For this review, use the dimensioned drawing (mm, ordinates from the lowest corner) and the shaded views. A direction names the side the tool comes from. Round coordinates to 2 decimals unless told otherwise and drop trailing zeros. Write each loop counter-clockwise with the first axis right and the second up, starting at its lowest first coordinate (ties: lowest second). Pieces come first, ordered by that corner, then holes.
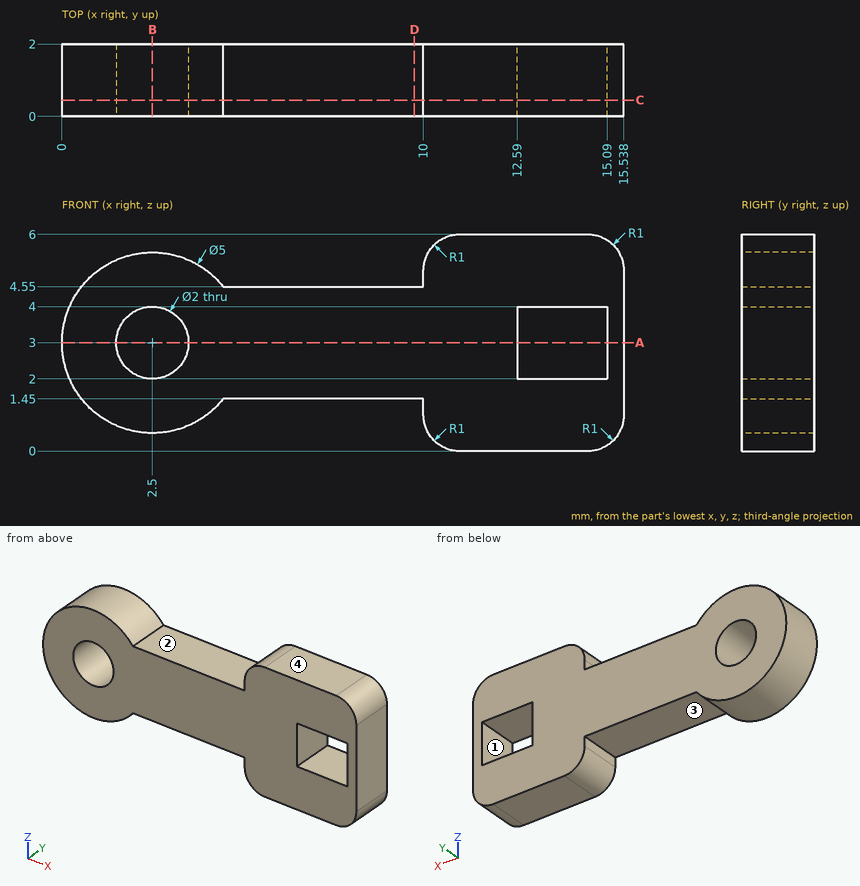
(1) We need section B-B, the plane x = 2.5. Give the boundary of the cut face in (y, z).
Geometry check:
outline: (0, 0.5) - (2, 0.5) - (2, 2) - (0, 2) - close; (0, 4) - (2, 4) - (2, 5.5) - (0, 5.5) - close
(2) For line 1 along X through (y, z) = (1.55, 3); line 2 along Z through (x, y) = (13, 0.5); line 3 along X through (y, z) = (1.75, 2.25) (1 decimal), list the stretches that pass through material, from the lowest coordinate up.
Geometry check:
line 1: x = 0 to 1.5, 3.5 to 12.59, 15.09 to 15.54
line 2: z = 0 to 2, 4 to 6
line 3: x = 0.1 to 1.8, 3.2 to 12.6, 15.1 to 15.5
(3) We need section D-D, the plane x = 9.75. Give the boundary of the cut face in (y, z).
Geometry check:
outline: (0, 1.45) - (2, 1.45) - (2, 4.55) - (0, 4.55) - close
(4) We need section C-C, the plane y = 0.45. Give the boundary of the cut face in (x, z).
Geometry check:
outline: (4.46, 1.45) - (10, 1.45) - (10, 1) arc R1 ccw to (11, 0) - (14.54, 0) arc R1 ccw to (15.54, 1) - (15.54, 5) arc R1 ccw to (14.54, 6) - (11, 6) arc R1 ccw to (10, 5) - (10, 4.55) - (4.46, 4.55) arc R2.5 ccw (long way) to start; hole circle Ø2 at (2.5, 3); hole (12.59, 2) - (15.09, 2) - (15.09, 4) - (12.59, 4) - close
(5) For pin 1 Ø1 at (x, y) = (7, 1) entering from -Z; pin 2 Ø1 at (x, y) = (8, 1) entering from +Z, all flat-tipped, find the tip position at first contact; note any pin that passes through.
Geometry check:
pin 1: stops at z = 1.45
pin 2: stops at z = 4.55
(6) For the marked faces 1, 2, 3 and 4, list the 3-axis set-ups (+Z, -Z, +X, -X, +Y, -Y) from which the entire face can be reached by the end or side of a thin tool; tool diameter is ignored.
Geometry check:
face 1: +Y, -Y
face 2: +Z, +Y, -Y
face 3: -Z, +Y, -Y
face 4: +Z, +X, -X, +Y, -Y
(7) We need section A-A, the plane z = 3. Give the boundary of the cut face in (x, y).
Geometry check:
outline: (0, 0) - (1.5, 0) - (1.5, 2) - (0, 2) - close; (3.5, 0) - (12.59, 0) - (12.59, 2) - (3.5, 2) - close; (15.09, 0) - (15.54, 0) - (15.54, 2) - (15.09, 2) - close
